from build123d import *

# Parameters (mm, degrees)
BOSS_EXTRUDE1_DEPTH = 10


with BuildPart() as part:
    # Sketch1 → Boss-Extrude1 (new body)
    with BuildSketch(Plane(origin=(0, 0, 0), x_dir=(-1, 0, 0), z_dir=(0, 0, -1))):
        Polygon((-15, 1.724031376), (-15, -10), (15, -10), (15, 10), (-6.724031376, 10), align=None)
    extrude(amount=-BOSS_EXTRUDE1_DEPTH)

    # Sketch2 → Revolve1 (revolve)
    with BuildSketch(Plane.XY.offset(5.2823368)):
        Polygon((18.993743672, 11.872423328), (17.9330835, 12.9330835), (10.862015688, 5.862015688), (11.92267586, 4.801355516), align=None)
    revolve(axis=Axis((18.463413586, 13.463413586, 5.2823368), (-0.7071067811865389, -0.7071067811865562, 0)))


solid = part.part
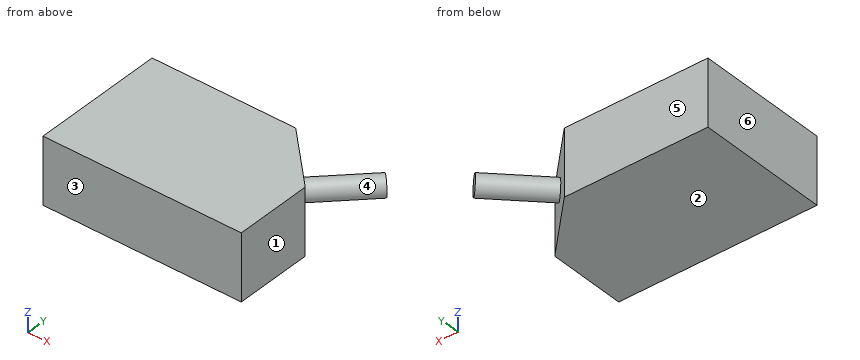
Can you work these out from the model? Positions are in its coordinate system, mm. Face numbers are marked on the shaded views. A direction names the side the tool comes from. Coordinates: 2 decimals unless noted, no trailing zeros. Order: outer loops, then holes, each group sorted by start corner. A loop starts at its lowest first (then second) coordinate and runs counter-clockwise, first axis right, second up. Notation, with made-up numbers: (79, -20) - (135, -20) arc R7 cw to (135, -12) - close; hole circle Ø8 at (-1.75, 31.5). An arc over 180 degrees is marked (long way). Answer as a JSON object with one key per item and string values. Group by question number.
Q1. Imagine slicing it at C-C (y = -4.75). Please give me the cut outline in (x, z).
Q2. We'd pull the mould along Y, two halves only. Please class the marked faces 3, 4, 5 and 6: +Y half, -Y half, draft (parallel to the pull), parting line (faces both ways), or undercut.
Q3. Imagine slicing it at B-B (x = 4.5). Please give me the cut outline in (y, z).
Q4. I need wall thicknesses on line 1 (X direction, y = -7.75, z = 7.75); line 2 (Y direction, x = -0.5, z = 7.5); line 3 (Y direction, x = 14, z = 4). Which ranges of each line are inside material? Lowest first, please. Write a range as from..to.
Q5. Will this pin go through, and if not, where does the flat tip stop? P1, Ø5, axis at x = 14.5, z = 3.5, coming from the +Y side.
Q6. Imagine slicing it at A-A (z = 8). Please give me the cut outline in (x, y).
Q7. Imagine slicing it at D-D (z = 5.75). Please give me the cut outline in (x, y), and give its area (3 significant figures).
Q8. On a 3-axis mill with a long thin cutter (end or side, diameter ignored), from which of +Z, -Z, +X, -X, +Y, -Y can I reach the whole of each face in a straight line? I mean the marked faces 1 and 2. Say none if no direction works.
Determined:
{
 "1": {"outline": "(-15, 0) - (15, 0) - (15, 10) - (-15, 10) - close"},
 "2": {"face 3": "-Y half", "face 4": "undercut", "face 5": "+Y half", "face 6": "draft"},
 "3": {"outline": "(-10, 0) - (10, 0) - (10, 10) - (-10, 10) - close"},
 "4": {"line 1": "x = -15..15", "line 2": "y = -10..10", "line 3": "y = -10..2.72, 7.9..10.1"},
 "5": {"P1": "stops at y = 13.65"},
 "6": {"outline": "(-15, -10) - (15, -10) - (15, 1.72) - (6.72, 10) - (-15, 10) - close"},
 "7": {"outline": "(-15, -10) - (15, -10) - (15, 1.72) - (11.87, 4.85) - (18.94, 11.93) - (16.93, 13.94) - (9.85, 6.87) - (6.72, 10) - (-15, 10) - close", "area": "594 mm2"},
 "8": {"face 1": "+Z, -Z, +X, -Y", "face 2": "-Z, +X, -X, +Y, -Y"}
}
